Model file for the job. Use its own axes, mm. Face numbers are marked on the shaded views. Round coordinates to 2 decimals unless told otherwise and drop trailing zeros. Loops run counter-clockwise (first coordinate to the right, second up) from the corner with the lowest first, then second, coordinate; pieces in that order, holes last. Notation, with made-up numbers: (82, 23.25) - (94, 23.25) arc R24 cw to (94, 39.25) - close; hole circle Ø2 at (-21, 25.5). An arc over 180 degrees is marked (long way). Answer as a JSON object with one key per item and string values.
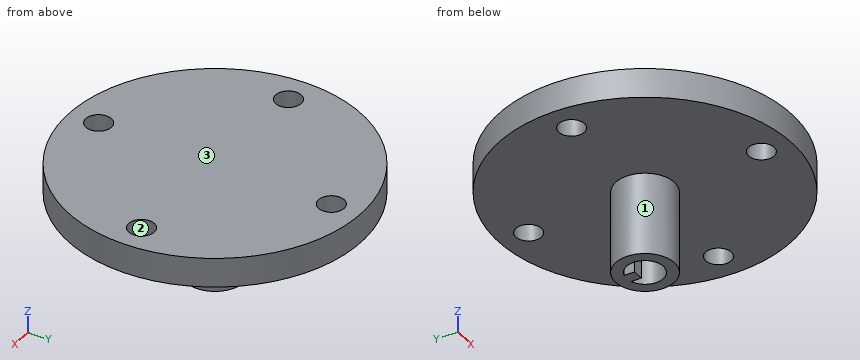
from build123d import *

# Parameters (mm, degrees)
SKETCH1_R           = 63.5
SKETCH1_R_2         = 5.55625
BOSS_EXTRUDE1_DEPTH = 12.7
SKETCH2_R           = 12.7
BOSS_EXTRUDE2_DEPTH = 35.56


with BuildPart() as part:
    # Sketch1 → Boss-Extrude1 (new body)
    with BuildSketch(Plane.XY):
        Circle(SKETCH1_R)
        with Locations((-50.8, 0)):
            Circle(SKETCH1_R_2, mode=Mode.SUBTRACT)
        with Locations((0, 50.8)):
            Circle(SKETCH1_R_2, mode=Mode.SUBTRACT)
        with Locations((50.8, 0)):
            Circle(SKETCH1_R_2, mode=Mode.SUBTRACT)
        with Locations((0, -50.8)):
            Circle(SKETCH1_R_2, mode=Mode.SUBTRACT)
    extrude(amount=BOSS_EXTRUDE1_DEPTH)

    # Sketch2 → Boss-Extrude2 (add)
    with BuildSketch(Plane(origin=(0, 0, 0), x_dir=(-1, 0, 0), z_dir=(0, 0, -1))):
        Circle(SKETCH2_R)
        with BuildLine():
            Line((-2.413, 7.561834252), (-2.413, 3.1115))
            Line((-2.413, 3.1115), (2.413, 3.1115))
            Line((2.413, 3.1115), (2.413, 7.561834252))
            ThreePointArc((2.413, 7.561834252), (0, -7.9375), (-2.413, 7.561834252))
        make_face(mode=Mode.SUBTRACT)
    extrude(amount=BOSS_EXTRUDE2_DEPTH)


solid = part.part
1) Two-plate mould, pull along X, no slides. Class the marked faces 1, 2 and 3: pulls with the +X half, pulls with the -X half, needs draft (parallel to the pull), parting line crosses it, or undercut.
Values follow:
{"face 1": "parting line crosses it", "face 2": "undercut", "face 3": "needs draft"}
2) Drop flat-ended pins along their axis: P1, Ø13, axis at x = 50.8, y = 0, coming from the -Z side; P2, Ø8, axis at x = 20, z = 5.5, coming from the +Y side; P3, Ø3.5, axis at y = 4.5, z = -15, coming from the -X side; P4, Ø9, axis at x = 0, y = 50.8, coming from the +Z side. Give the stop position or say it passes through.
Values follow:
{"P1": "z = 0", "P2": "y = 61.45", "P3": "x = -12.4", "P4": "through"}
3) Slice it at D-D on x = 0. List the corners of the cut face in (y, z), then the cut area to 3 significant figures.
Values follow:
{"outline": "(-63.5, 0) - (-56.36, 0) - (-56.36, 12.7) - (-63.5, 12.7) - close; (-45.24, 0) - (-12.7, 0) - (-12.7, -35.56) - (-7.94, -35.56) - (-7.94, 0) - (3.11, 0) - (3.11, -35.56) - (12.7, -35.56) - (12.7, 0) - (45.24, 0) - (45.24, 12.7) - (-45.24, 12.7) - close; (56.36, 0) - (63.5, 0) - (63.5, 12.7) - (56.36, 12.7) - close", "area": "1,840 mm²"}
4) Slice it at A-A on x = -50.8. List the corners of the cut face in (y, z).
Values follow:
{"outline": "(-38.1, 0) - (-5.56, 0) - (-5.56, 12.7) - (-38.1, 12.7) - close; (5.56, 0) - (38.1, 0) - (38.1, 12.7) - (5.56, 12.7) - close"}
5) Slice it at C-C on z = -15.5. List the corners of the cut face in (x, y) (1 decimal), then the cut area to 3 significant figures.
Values follow:
{"outline": "circle Ø25.4 at (0, 0); hole (-2.4, 3.1) - (-2.4, 7.6) arc R7.9 ccw (long way) to (2.4, 7.6) - (2.4, 3.1) - close", "area": "331 mm²"}
6) Probe probe 1 along Y at (x, z) = (0, 5); probe 2 along Y at (x, z) = (0, -16.5); probe 3 along Z at (x, y) = (41.5, 19). List the from-to ranges inside material, lowest first.
Values follow:
{"probe 1": "-63.5 to -56.36, -45.24 to 45.24, 56.36 to 63.5", "probe 2": "-12.7 to -7.94, 3.11 to 12.7", "probe 3": "0 to 12.7"}
